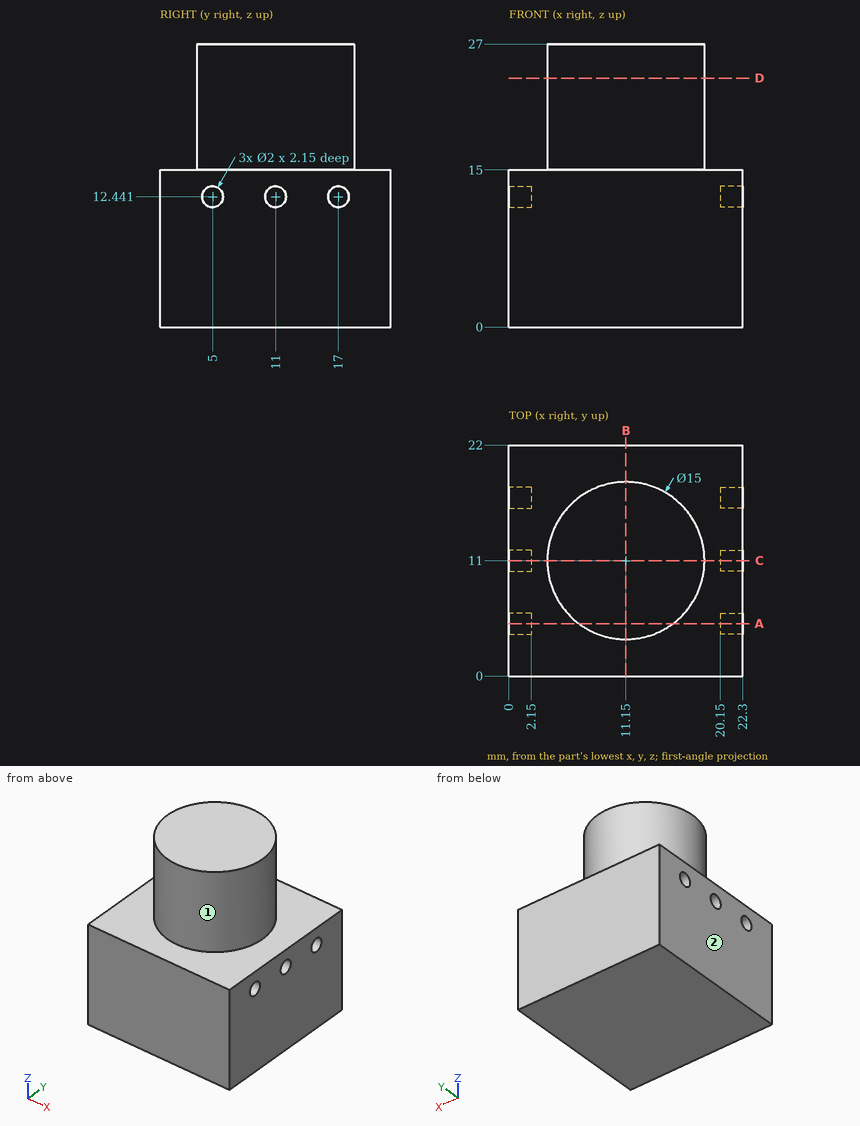
Answer from the drawing. Dimensions are ordinates in mm from the lowest x, y and z of the part. A direction names the side the tool comes from. Coordinates: 2 decimals unless noted, no trailing zeros. Write each loop counter-clockwise with the first axis right and the second up, starting at its lowest first coordinate (ties: lowest second). Pieces come first, ordered by that corner, then holes. Notation, with made-up numbers: M 76.25,27.25 L 103.25,27.25 A10 cw 103.25,45.25 Z; hole C -0.5,-21.5 d6. An arc over 180 degrees is marked long. Put each result on its own line as item: value. Start each with the question number.
1. Consider line 1 (Z direction, x = 0.75, y = 17); line 2 (Z direction, x = 19.25, y = 3.5); line 3 (X direction, y = 10.75, z = 16). Determine where each line is inside the solid, lowest interval first. Write a range as from..to.
2. A cutting plane is placed at B-B on x = 11.15. Write down the section's boundary in (y, z).
3. Which of the six approach directions +Z, -Z, +X, -X, +Y, -Y give full straight-line access (tool end or side, diameter ignored) to the marked faces 1 and 2?
4. Flat-ended cylindrical pins translate along their axes: P1, Ø1.8, axis at y = 5, z = 12.44, coming from the +X side; P2, Ø1, axis at y = 15, z = 24, coming from the +X side; P3, Ø4, axis at x = 3.5, y = 18, coming from the +Z side. Find the tip coordinate at first contact, or state that the pin passes through.
5. A cutting plane is placed at A-A on y = 5. Write down the section's boundary in (x, z), then the cut area to 3 significant figures.
6. A cutting plane is placed at D-D on z = 23.75. Write down the section's boundary in (x, y).
7. A cutting plane is placed at C-C on y = 11. Write down the section's boundary in (x, z), then the cut area to 3 significant figures.
Resolved:
1. line 1: z = 0..11.44, 13.44..15
1. line 2: z = 0..15
1. line 3: x = 3.65..18.65
2. outline: M 0,0 L 22,0 L 22,15 L 18.5,15 L 18.5,27 L 3.5,27 L 3.5,15 L 0,15 Z
3. face 1: +Z
3. face 2: +Z, -Z, -X, +Y, -Y
4. P1: stops at x = 20.15
4. P2: stops at x = 17.78
4. P3: stops at z = 15
5. outline: M 0,0 L 22.3,0 L 22.3,11.44 L 20.15,11.44 L 20.15,13.44 L 22.3,13.44 L 22.3,15 L 15.65,15 L 15.65,27 L 6.65,27 L 6.65,15 L 0,15 L 0,13.44 L 2.15,13.44 L 2.15,11.44 L 0,11.44 Z
5. area: 434 mm2
6. outline: C 11.15,11 d15
7. outline: M 0,0 L 22.3,0 L 22.3,11.44 L 20.15,11.44 L 20.15,13.44 L 22.3,13.44 L 22.3,15 L 18.65,15 L 18.65,27 L 3.65,27 L 3.65,15 L 0,15 L 0,13.44 L 2.15,13.44 L 2.15,11.44 L 0,11.44 Z
7. area: 506 mm2
